```python
from build123d import *

# Parameters (mm, degrees)
SKETCH1_W           = 170
SKETCH1_H           = 130
BOSS_EXTRUDE1_DEPTH = 5
SKETCH3_R           = 1.75
CUT_EXTRUDE1_DEPTH  = 108.121426428
SKETCH4_R           = 1.55
SKETCH4_R_2         = 1.6
SKETCH4_R_3         = 1.5
CUT_EXTRUDE2_DEPTH  = 108.121426428
CUT_EXTRUDE3_DEPTH  = 108.121426428
CUT_EXTRUDE4_DEPTH  = 108.121426428
FILLET1_R           = 15
SKETCH7_R           = 1.6
CUT_EXTRUDE5_DEPTH  = 10


with BuildPart() as part:
    # Sketch1 → Boss-Extrude1 (new body)
    with BuildSketch(Plane(origin=(0, 0, 0), x_dir=(1, 0, 0), z_dir=(0, 1, 0))):
        Rectangle(SKETCH1_W, SKETCH1_H)
    extrude(amount=BOSS_EXTRUDE1_DEPTH)

    # Sketch3 → Cut-Extrude1 (cut, through all)
    with BuildSketch(Plane(origin=(0, 5, 0), x_dir=(1, 0, 0), z_dir=(0, 1, 0))):
        with Locations(Location((41.55, 56.25, 0), (0, 0, 270))):
            Circle(SKETCH3_R)
        with Locations(Location((71.55, 56.25, 0), (0, 0, 270))):
            Circle(SKETCH3_R)
        with Locations(Location((71.55, 33, 0), (0, 0, 270))):
            Circle(SKETCH3_R)
        with Locations(Location((41.55, 33, 0), (0, 0, 270))):
            Circle(SKETCH3_R)
        with Locations(Location((41.55, -33, 0), (0, 0, 90))):
            Circle(SKETCH3_R)
        with Locations(Location((71.55, -33, 0), (0, 0, 90))):
            Circle(SKETCH3_R)
        with Locations(Location((71.55, -56.25, 0), (0, 0, 90))):
            Circle(SKETCH3_R)
        with Locations(Location((41.55, -56.25, 0), (0, 0, 90))):
            Circle(SKETCH3_R)
        with Locations(Location((-41.55, -56.25, 0), (0, 0, 270))):
            Circle(SKETCH3_R)
        with Locations(Location((-71.55, -56.25, 0), (0, 0, 270))):
            Circle(SKETCH3_R)
        with Locations(Location((-71.55, -33, 0), (0, 0, 270))):
            Circle(SKETCH3_R)
        with Locations(Location((-41.55, -33, 0), (0, 0, 270))):
            Circle(SKETCH3_R)
        with Locations(Location((-41.55, 33, 0), (0, 0, 90))):
            Circle(SKETCH3_R)
        with Locations(Location((-71.55, 33, 0), (0, 0, 90))):
            Circle(SKETCH3_R)
        with Locations(Location((-71.55, 56.25, 0), (0, 0, 90))):
            Circle(SKETCH3_R)
        with Locations(Location((-41.55, 56.25, 0), (0, 0, 90))):
            Circle(SKETCH3_R)
    extrude(amount=-CUT_EXTRUDE1_DEPTH, mode=Mode.SUBTRACT)

    # Sketch4 → Cut-Extrude2 (cut, through all)
    with BuildSketch(Plane.XZ):
        with Locations(Location((78.25, -19.55, 0), (0, 0, 270))):
            Circle(SKETCH4_R)
        with Locations(Location((41.55, -19.55, 0), (0, 0, 270))):
            Circle(SKETCH4_R)
        with Locations(Location((78.25, -56.25, 0), (0, 0, 270))):
            Circle(SKETCH4_R)
        with Locations(Location((78.25, 56.25, 0), (0, 0, 270))):
            Circle(SKETCH4_R)
        with Locations(Location((78.25, 19.55, 0), (0, 0, 270))):
            Circle(SKETCH4_R)
        with Locations(Location((41.55, 19.55, 0), (0, 0, 270))):
            Circle(SKETCH4_R)
        with Locations(Location((-17.7, 59.3, 0), (0, 0, 270))):
            Circle(SKETCH4_R_2)
        with Locations(Location((17.7, 40.7, 0), (0, 0, 270))):
            Circle(SKETCH4_R_2)
        with Locations(Location((4.5, 10.5, 0), (0, 0, 270))):
            Circle(SKETCH4_R_3)
        with Locations(Location((4.5, -10.5, 0), (0, 0, 270))):
            Circle(SKETCH4_R_3)
        with Locations(Location((15.5, -41.5, 0), (0, 0, 270))):
            Circle(SKETCH4_R_3)
        with Locations(Location((15.5, -62.5, 0), (0, 0, 270))):
            Circle(SKETCH4_R_3)
        with Locations(Location((-15.5, -41.5, 0), (0, 0, 270))):
            Circle(SKETCH4_R_3)
        with Locations(Location((-15.5, -62.5, 0), (0, 0, 270))):
            Circle(SKETCH4_R_3)
    extrude(amount=-CUT_EXTRUDE2_DEPTH, mode=Mode.SUBTRACT)

    # Sketch5 → Cut-Extrude3 (cut, through all)
    with BuildSketch(Plane(origin=(0, 5, 0), x_dir=(1, 0, 0), z_dir=(0, 1, 0))):
        with BuildLine():
            Line((62, 7), (37, 7))
            ThreePointArc((37, 7), (30, 0), (37, -7))
            Line((37, -7), (62, -7))
            ThreePointArc((62, -7), (69, 0), (62, 7))
        make_face()
    extrude(amount=-CUT_EXTRUDE3_DEPTH, mode=Mode.SUBTRACT)

    # Sketch6 → Cut-Extrude4 (cut, through all)
    with BuildSketch(Plane(origin=(0, 5, 0), x_dir=(1, 0, 0), z_dir=(0, 1, 0))):
        with BuildLine():
            ThreePointArc((-75, 0), (-77.928932188, 7.071067812), (-85, 10))
            Line((-85, 10), (-85, -10))
            ThreePointArc((-85, -10), (-77.928932188, -7.071067812), (-75, 0))
        make_face()
        with BuildLine():
            Line((-85, -10), (-85, 10))
            ThreePointArc((-85, 10), (-95, 0), (-85, -10))
        make_face()
    extrude(amount=-CUT_EXTRUDE4_DEPTH, mode=Mode.SUBTRACT)

    # Fillet1
    fillet1_edges = [part.edges().sort_by_distance(p)[0] for p in [
        (85, 2.5, 65),
        (-85, 2.5, 65),
        (-85, 2.5, -65),
        (85, 2.5, -65),
    ]]
    fillet(fillet1_edges, radius=FILLET1_R)

    # Sketch7 → Cut-Extrude5 (cut)
    with BuildSketch(Plane(origin=(0, 5, 0), x_dir=(1, 0, 0), z_dir=(0, 1, 0))):
        with Locations(Location((20, 0, 0), (0, 0, 270))):
            Circle(SKETCH7_R)
        with Locations(Location((-20, 0, 0), (0, 0, 270))):
            Circle(SKETCH7_R)
    extrude(amount=-CUT_EXTRUDE5_DEPTH, mode=Mode.SUBTRACT)


solid = part.part
```
Read the model definition and answer for the solid it produces. Units are mm, in the model's axes. A direction names the side the tool comes from. Coordinates: 2 decimals unless noted, no trailing zeros. Loops run counter-clockwise (first coordinate to the right, second up) from the corner with the lowest first, then second, coordinate; pieces in that order, holes last. Notation, with made-up numbers: (67.25, 31) -> (115.25, 31) arc R25 cw to (115.25, 47) -> close; hole circle Ø6 at (7, -29.5). An arc over 180 degrees is marked (long way). Return JSON: item names as keys, results as strings.
Item 1: Find section B-B (y = 3.4). Count the separate pieces of the cut face and the enclosed holes in it, plus the area to 3 significant figures.
Answers:
{"separate pieces": "1", "enclosed holes": "33", "area": "21,000 mm2"}
Item 2: For a pull along Z with two mould halves and no side action, classify faces 3 (the cylindrical face through (-80.72, 2.54, 60.49)), 4 (the cylindrical face through (72.22, 2.535, 54.633)), 5 (the flat face through (85, 2, 1)) as +Z half, -Z half, draft (parallel to the pull), parting line (faces both ways), or undercut.
Answers:
{"face 3": "+Z half", "face 4": "undercut", "face 5": "draft"}
Item 3: Find the intervals of material crossed by probe 1 along X at (y, z) = (1.3, -33); probe 2 along Z at (x, y) = (71.55, 1.55); probe 3 along X at (y, z) = (1.85, -41.5), in increasing order.
Answers:
{"probe 1": "x = -85 to -73.3, -69.8 to -43.3, -39.8 to 39.8, 43.3 to 69.8, 73.3 to 85", "probe 2": "z = -64.92 to -58, -54.5 to -34.75, -31.25 to 31.25, 34.75 to 54.5, 58 to 64.92", "probe 3": "x = -85 to -17, -14 to 14, 17 to 85"}
Item 4: For faces 1 (the cylindrical face through (69, 3, 0)), 2 (the flat face through (-85, 2, 30)), determine the directions among +Z, -Z, +X, -X, +Y, -Y from which every point of the face is accessible in a straight line to the end or side of a thin tool.
Answers:
{"face 1": "+Y, -Y", "face 2": "+Z, -Z, -X, +Y, -Y"}
Item 5: Find section A-A (x = 60). Determine the outline of the cut face in (y, z), plus the area to 3 significant figures.
Answers:
{"outline": "(0, -65) -> (5, -65) -> (5, -7) -> (0, -7) -> close; (0, 7) -> (5, 7) -> (5, 65) -> (0, 65) -> close", "area": "580 mm2"}
